Part model, mm, in its own coordinate system. Face numbers are marked on the shaded views. A direction names the side the tool comes from. Round coordinates to 2 decimals unless told otherwise and drop trailing zeros. Loops run counter-clockwise (first coordinate to the right, second up) from the corner with the lowest first, then second, coordinate; pieces in that order, holes last.
1) Band-saw the part on D-D, the plane x = 8.5. Write the cut outline in (y, z), then the cut area to 3 significant figures.
2) Band-saw the part on B-B, the plane z = 4.3. Write the cut outline in (x, y), then the cut area to 3 significant figures.
3) Probe line 1 (X direction, y = 1.45, z = 4.3); line 2 (X direction, y = 3.25, z = 6); line 3 (Y direction, x = 3.5, z = 2.5). List the from-to ranges inside material, lowest first.
4) Mould opens along X. For the marked faces 1, 2 and 3 say: +X half, -X half, draft (parallel to the pull), parting line (faces both ways), or undercut.
5) Band-saw the part on A-A, the plane y = 2.5. Write the cut outline in (x, z), then the cut area to 3 significant figures.
6) Drop flat-ended pins along their axis: P1, Ø2, axis at x = -9, z = 4.3, coming from the +Y side; P2, Ø3.5, axis at y = 6, z = 8, coming from the -X side; P3, Ø0.9, axis at x = -8, y = 1.5, coming from the +Z side; P4, Ø4, axis at x = 0.5, z = 10, coming from the -Y side. Give the stop position or say it passes through.
7) Band-saw the part on C-C, the plane y = 5.5. Write the cut outline in (x, z), then the cut area to 3 significant figures.
8) 3-axis set-ups, long thin cutter, end or side, ignore diameter. For the marked faces 4, 5 and 6: which of +Z, -Z, +X, -X, +Y, -Y reach the whole face in a straight line?
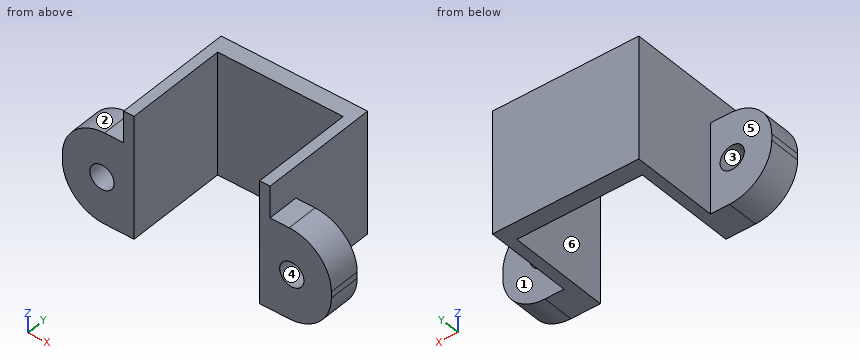
Autodesk Inventor part; units mm, degrees
ref_plane "YZ Plane" through (0, 0, 0) normal (1, 0, 0) x (0, 1, 0)
ref_plane "XZ Plane" through (0, 0, 0) normal (0, 1, 0) x (-1, 0, 0)
ref_plane "XY Plane" through (0, 0, 0) normal (0, 0, 1) x (1, 0, 0)
sketch "Sketch1" plane through (0, 0, 0) normal (0, 0, 1) x (1, 0, 0)
  line L0 (0, 0) -> (12.75, 0)
  line L1 (0, 0) -> (-12.75, 0)
  line L2 (-12.75, 0) -> (-12.75, 11.32)
  line L3 (-12.75, 11.32) -> (12.75, 11.32)
  line L4 (12.75, 11.32) -> (12.75, 0)
  line L5 (0, 0) -> (-5.95, 0)
  line L6 (0, 0) -> (5.95, 0)
  line L7 (12.75, 0) -> (6.94, 0)
  line L8 (0, 11.32) -> (0, 9.7)
  line L9 (0, 9.7) -> (6.94, 9.7)
  line L10 (6.94, 9.7) -> (6.94, 0)
  line L11 (0, 0) -> (0, 11.32)
  line L12 (0, 9.7) -> (-6.94, 9.7)
  line L13 (-6.94, 9.7) -> (-6.94, 0)
  line L14 (-12.75, 0) -> (-6.94, 0)
  line L15 (12.75, 0) -> (12.75, 3)
  line L16 (12.75, 3) -> (6.94, 3)
  line L17 (-12.75, 3) -> (-6.94, 3)
  line L18 (-6.94, 9.7) -> (-6.94, 11.32)
  line L19 (6.94, 9.7) -> (6.94, 11.32)
  line L20 (5.95, 0) -> (5.95, 9.7)
  line L21 (-5.95, 0) -> (-5.95, 9.7)
  dimension "d0" = 12.75
  dimension "d1" = 12.75
  dimension "d2" = 11.32
  dimension "d3" = 25.5
  dimension "d4" = 5.95
  dimension "d5" = 5.95
  dimension "d6" = 5.81
  dimension "d7" = 1.62
  dimension "d8" = 5.81
  dimension "d9" = 3
extrude "Extrusion1" add sketch "Sketch1" along normal blind 11.6 contours L20 L9 L10 L0 | L1 L13 L12 L21 | L12 L18 L3 L8 | L8 L3 L19 L9 | L10 L16 L4 L0 | L1 L2 L17 L13
sketch "Sketch2" plane through (6.94, 3, 0) normal (0, 1, 0) x (1, 0, 0)
  line L0 (-6.94, 0) -> (-6.94, -11.6)
  line L1 (-12.89, -11.6) -> (-0.99, -11.6)
  line L2 (-0.99, -11.6) -> (5.81, -11.6)
  line L3 (5.81, -11.6) -> (5.81, -8.6)
  line L4 (5.81, -8.6) -> (0, -8.6)
  line L5 (0, 0) -> (0, -11.6)
  line L6 (0, -11.6) -> (5.81, -11.6)
  line L7 (2.905, -8.6) -> (2.905, 0)
  line L8 (-0.99, 0) -> (5.81, 0)
  line L9 (5.81, 0) -> (5.81, -11.6)
  line L10 (5.81, -8.6) -> (5.81, 0)
  line L11 (-12.89, -11.6) -> (-19.69, -11.6)
  line L12 (-19.69, -11.6) -> (-19.69, -8.6)
  line L13 (-19.69, -8.6) -> (-13.88, -8.6)
  line L14 (-13.88, 0) -> (-13.88, -11.6)
  line L15 (-16.785, -8.6) -> (-16.785, 0)
  dimension "d12" = 3
extrude "Extrusion2" cut sketch "Sketch2" against normal blind 11.6 contours L5 L4 L3 L2 | L11 L12 L13 L14
fillet "Fillet1" radius 4 4 edges at (-12.75, 1.5, 0) (-12.75, 1.5, 8.6) (12.75, 1.5, 0) (12.75, 1.5, 8.6)
sketch "Sketch4" plane through (6.94, 3, 8.6) normal (0, 1, 0) x (1, 0, 0)
  line L0 (5.81, 4.6) -> (5.81, 4)
  line L1 (5.81, 4.3) -> (-19.69, 4.3)
  line L2 (-19.69, 4.6) -> (-19.69, 4)
  line L3 (-6.94, 8.6) -> (-6.94, 4.3)
  line L4 (-6.94, 4.3) -> (2.06, 4.3)
  line L5 (-6.94, 4.3) -> (-15.94, 4.3)
  circle A0 centre (-15.94, 4.3) radius 1.15
  circle A1 centre (2.06, 4.3) radius 1.15
  dimension "d16" = 9
  dimension "d17" = 9
  dimension "d18" = 2.3
  dimension "d19" = 2.3
extrude "Extrusion3" cut sketch "Sketch4" against normal blind 11.6
properties part number "SoporteMotor_3.0"
Reported:
1. outline: (0, 0) - (3, 0) - (3, 3.26) - (0, 3.26) - close; (0, 5.34) - (3, 5.34) - (3, 8.6) - (0, 8.6) - close
1. area: 19.6 mm2
2. outline: (-12.75, 0) - (-10.15, 0) - (-10.15, 3) - (-12.75, 3) - close; (-7.85, 0) - (-5.95, 0) - (-5.95, 9.7) - (5.95, 9.7) - (5.95, 0) - (7.85, 0) - (7.85, 3) - (6.94, 3) - (6.94, 11.32) - (-6.94, 11.32) - (-6.94, 3) - (-7.85, 3) - close; (10.15, 0) - (12.75, 0) - (12.75, 3) - (10.15, 3) - close
2. area: 62.8 mm2
3. line 1: x = -12.75 to -10.15, -7.85 to -5.95, 5.95 to 7.85, 10.15 to 12.75
3. line 2: x = -6.94 to -5.95, 5.95 to 6.94
3. line 3: y = 9.7 to 11.32
4. face 1: draft
4. face 2: -X half
4. face 3: undercut
5. outline: (-12.75, 4) arc R4 ccw to (-8.75, 0) - (-5.95, 0) - (-5.95, 11.6) - (-6.94, 11.6) - (-6.94, 8.6) - (-8.75, 8.6) arc R4 ccw to (-12.75, 4.6) - close; (5.95, 0) - (8.75, 0) arc R4 ccw to (12.75, 4) - (12.75, 4.6) arc R4 ccw to (8.75, 8.6) - (6.94, 8.6) - (6.94, 11.6) - (5.95, 11.6) - close; hole circle Ø2.3 at (-9, 4.3); hole circle Ø2.3 at (9, 4.3)
5. area: 101 mm2
6. P1: passes through
6. P2: stops at x = -6.94
6. P3: stops at z = 8.6
6. P4: stops at y = 9.7
7. outline: (-6.94, 0) - (-5.95, 0) - (-5.95, 11.6) - (-6.94, 11.6) - close; (5.95, 0) - (6.94, 0) - (6.94, 11.6) - (5.95, 11.6) - close
7. area: 23.0 mm2
8. face 4: +Y, -Y
8. face 5: +Z, -Z, -X, +Y
8. face 6: +Z, -Z, -Y
